```python
from build123d import *

# Parameters (mm, degrees)
SKETCH1_R                 = 82.2325
SKETCH1_R_2               = 68.2625
SKETCH1_R_3               = 1.1303
SKETCH1_R_4               = 1.3589
BOSS_EXTRUDE1_DEPTH       = 7.62
BOSS_EXTRUDE3_START       = 7.62
SKETCH1_3_R               = 82.2325
SKETCH1_3_R_2             = 1.1303
SKETCH1_3_R_3             = 75.2475
BOSS_EXTRUDE3_DEPTH       = 8.636
CIRPATTERN1_OUTLINE_R     = 1.1303
CIRPATTERN1_DEPTH         = 16.256
SKETCH2_R                 = 1.651
SKETCH1_4_R               = 5.588
SKETCH1_4_R_2             = 1.9939
CUT_EXTRUDE2_DEPTH        = 0.635
SKETCH1_5_R               = 1.9939
CUT_EXTRUDE3_DEPTH        = 6.35
CIRPATTERN3_OUTLINE_R     = 1.3589
CIRPATTERN3_OUTLINE_R_2   = 1.9939
CIRPATTERN3_DEPTH         = 6.35
CIRPATTERN3_2_OUTLINE_R   = 5.588
CIRPATTERN3_2_OUTLINE_R_2 = 1.9939
CIRPATTERN3_2_DEPTH       = 0.635
CIRPATTERN3_START         = 6.35
CIRPATTERN3_3_OUTLINE_R   = 1.3589
CIRPATTERN3_3_DEPTH       = 1.27


# Read off the part's stored shape, not the designer's step: CirPattern1, CirPattern3
with BuildPart() as part:
    # Sketch1 → Boss-Extrude1 (new body)
    with BuildSketch(Plane(origin=(0, 0, 0), x_dir=(1, 0, 0), z_dir=(0, 1, 0))):
        with Locations(Location((0, 0, 0), (0, 0, 90))):
            Circle(SKETCH1_R)
        with Locations(Location((0, 0, 0), (0, 0, 90))):
            Circle(SKETCH1_R_2, mode=Mode.SUBTRACT)
        with Locations(Location((0, -78.74, 0), (0, 0, 90))):
            Circle(SKETCH1_R_3, mode=Mode.SUBTRACT)
        with Locations(Location((61.639143453, -43.160192894, 0), (0, 0, 90))):
            Circle(SKETCH1_R_4, mode=Mode.SUBTRACT)
    extrude(amount=BOSS_EXTRUDE1_DEPTH)

    # Sketch1<3> → Boss-Extrude3 (add)
    with BuildSketch(Plane(origin=(0, 0, 0), x_dir=(1, 0, 0), z_dir=(0, 1, 0)).offset(BOSS_EXTRUDE3_START)):
        with Locations(Location((0, 0, 0), (0, 0, 90))):
            Circle(SKETCH1_3_R)
        with Locations(Location((0, -78.74, 0), (0, 0, 90))):
            Circle(SKETCH1_3_R_2, mode=Mode.SUBTRACT)
        with Locations(Location((0, 0, 0), (0, 0, 326.034722653))):
            Circle(SKETCH1_3_R_3, mode=Mode.SUBTRACT)
    extrude(amount=BOSS_EXTRUDE3_DEPTH)

    # CirPattern1 outline → CirPattern1 (cut)
    with BuildSketch(Plane(origin=(0, 0, 0), x_dir=(1, 0, 0), z_dir=(0, 1, 0))):
        with Locations((-68.190840294, -39.37)):
            Circle(CIRPATTERN1_OUTLINE_R)
        with Locations((-68.190840294, 39.37)):
            Circle(CIRPATTERN1_OUTLINE_R)
        with Locations((0, 78.74)):
            Circle(CIRPATTERN1_OUTLINE_R)
        with Locations((68.190840294, 39.37)):
            Circle(CIRPATTERN1_OUTLINE_R)
        with Locations((68.190840294, -39.37)):
            Circle(CIRPATTERN1_OUTLINE_R)
    extrude(amount=CIRPATTERN1_DEPTH, mode=Mode.SUBTRACT)

    # Sketch2 → Cut-Revolve2 (revolve, cut)
    with BuildSketch(Plane(origin=(0, 0, 0), x_dir=(0, 0, -1), z_dir=(1, 0, 0))):
        with Locations((71.755, 8.509)):
            Circle(SKETCH2_R)
    revolve(axis=Axis((0, 7.62, 0), (0, 1, 0)), mode=Mode.SUBTRACT)

    # Sketch1<4> → Cut-Extrude2 (cut)
    with BuildSketch(Plane(origin=(0, 0, 0), x_dir=(1, 0, 0), z_dir=(0, 1, 0))):
        with Locations(Location((36.98875, -64.066394308, 0), (0, 0, 270))):
            Circle(SKETCH1_4_R)
        with Locations(Location((36.98875, -64.066394308, 0), (0, 0, 270))):
            Circle(SKETCH1_4_R_2, mode=Mode.SUBTRACT)
    extrude(amount=CUT_EXTRUDE2_DEPTH, mode=Mode.SUBTRACT)

    # Sketch1<5> → Cut-Extrude3 (cut)
    with BuildSketch(Plane(origin=(0, 0, 0), x_dir=(1, 0, 0), z_dir=(0, 1, 0))):
        with Locations(Location((36.98875, -64.066394308, 0), (0, 0, 270))):
            Circle(SKETCH1_5_R)
    extrude(amount=CUT_EXTRUDE3_DEPTH, mode=Mode.SUBTRACT)

    # CirPattern3 outline → CirPattern3 (cut)
    with BuildSketch(Plane(origin=(0, 0, 0), x_dir=(1, 0, 0), z_dir=(0, 1, 0))):
        with Locations((-68.197395205, -31.80096765)):
            Circle(CIRPATTERN3_OUTLINE_R)
        with Locations((6.558251752, 74.961160545)):
            Circle(CIRPATTERN3_OUTLINE_R)
        with Locations((36.98875, 64.066394308)):
            Circle(CIRPATTERN3_OUTLINE_R_2)
        with Locations((-73.9775, 0)):
            Circle(CIRPATTERN3_OUTLINE_R_2)
    extrude(amount=CIRPATTERN3_DEPTH, mode=Mode.SUBTRACT)

    # CirPattern3 2 outline → CirPattern3 2 (cut)
    # profile 1 of 2: a face of its own
    with BuildSketch(Plane(origin=(0, 0, 0), x_dir=(1, 0, 0), z_dir=(0, 1, 0))):
        with Locations((-73.9775, 0)):
            Circle(CIRPATTERN3_2_OUTLINE_R)
        with Locations((-73.9775, 0)):
            Circle(CIRPATTERN3_2_OUTLINE_R_2, mode=Mode.SUBTRACT)
    # profile 2 of 2: a face of its own
    with BuildSketch(Plane(origin=(0, 0, 0), x_dir=(1, 0, 0), z_dir=(0, 1, 0))):
        with Locations((36.98875, 64.066394308)):
            Circle(CIRPATTERN3_2_OUTLINE_R)
        with Locations((36.98875, 64.066394308)):
            Circle(CIRPATTERN3_2_OUTLINE_R_2, mode=Mode.SUBTRACT)
    extrude(amount=CIRPATTERN3_2_DEPTH, mode=Mode.SUBTRACT)

    # CirPattern3 3 outline → CirPattern3 3 (cut)
    with BuildSketch(Plane(origin=(0, 0, 0), x_dir=(1, 0, 0), z_dir=(0, 1, 0)).offset(CIRPATTERN3_START)):
        with Locations((-68.197395205, -31.80096765)):
            Circle(CIRPATTERN3_3_OUTLINE_R)
        with Locations((6.558251752, 74.961160545)):
            Circle(CIRPATTERN3_3_OUTLINE_R)
    extrude(amount=CIRPATTERN3_3_DEPTH, mode=Mode.SUBTRACT)


solid = part.part
```
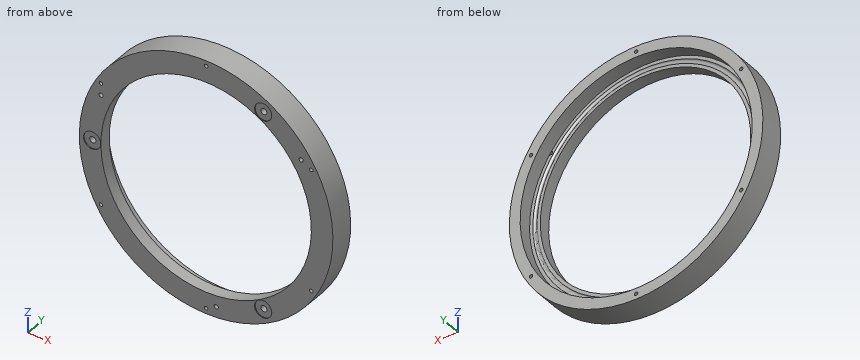
Geometry check sheet. Reference: the model listing, model coordinates, mm. Coordinates: 2 decimals unless noted, no trailing zeros. Write each loop counter-clockwise with the first axis right and the second up, starting at its lowest first coordinate (ties: lowest second). Pieces come first, ordered by that corner, then holes. Notation, with made-up numbers: M 67,35 L 77,35 A12 ccw 77,52 Z; hole C 68,66.25 d10. An arc over 180 degrees is marked long. Answer as a JSON object with one key per item and string values.
1. Section check A-A, the plane y = 13.25. Enter the section's corners in (x, z) (1 decimal), plus the area to 3 significant figures.
Answers below:
{"outline": "C 0,0 d164.5; hole C 0,0 d150.5; hole C -68.2,-39.4 d2.3; hole C -68.2,39.4 d2.3; hole C 0,-78.7 d2.3; hole C 0,78.7 d2.3; hole C 68.2,-39.4 d2.3; hole C 68.2,39.4 d2.3", "area": "3,430 mm²"}
2. Scan lines: L1, parallel to X at y = 7.5, z = -12; L2, parallel to Z at x = -49.5, y = 8.5; L3, parallel to Y at x = -20.5, z = 72. Record each from-to range of solid material in increasing order.
Answers below:
{"L1": "x = -81.35 to -72.07, -69.42 to -67.2, 67.2 to 69.42, 72.07 to 81.35", "L2": "z = -65.67 to -56.67, 56.67 to 65.67", "L3": "y = 0 to 7.62"}
3. Go/stop test with flat-tipped pins: pin 1 Ø1.5 at (x, y) = (-58, 4) entering from -Z; pin 2 Ø4.5 at (x, z) = (37.5, -63.5) entering from -Y (3 decimals); pin 3 Ø3 at (x, z) = (68.19, -39.37) entering from -Y; pin 4 Ø6 at (x, y) = (-18, 3) entering from +Z. Record where each tip stops, or that it passes through.
Answers below:
{"pin 1": "stops at z = -59.03", "pin 2": "stops at y = 0.635", "pin 3": "stops at y = 0", "pin 4": "stops at z = 80.85"}
